Work out the finished part from the listing and answer in its coordinate system (mm). A direction names the side the tool comes from. Coordinates: 2 decimals unless noted, no trailing zeros. Write each loop counter-clockwise with the first axis right and the second up, starting at its lowest first coordinate (ties: lowest second). Pieces come first, ordered by that corner, then holes. Notation, with made-up numbers: M 77,27 L 100,27 A31 ccw 100,65 Z; hole C 78.25,63 d8. An arc over 180 degrees is marked long. Use CSV: the item, a comma, the result in double quotes.
from build123d import *

# Parameters (mm, degrees)
F1_R     = 6.15
F2_DEPTH = 35.5
F3_DEPTH = 35.501
F4_DEPTH = 2
F5_R     = 0.5


# Not quite as in the source:
# - two fillets or chamfers of one size are made in one step


with BuildPart() as f2:
    # F1 (on face) → F2 (new body)
    with BuildSketch(Plane.XZ):
        Circle(F1_R)
    extrude(amount=F2_DEPTH)


with BuildPart() as f2b:
    # F0 (on Front) → F2, piece 2 (new body)
    with BuildSketch(Plane.XZ):
        with BuildLine():
            ThreePointArc((11.8124997243, -2.1130192291), (11.9530330187, -1.0606609515), (12, 0))
            ThreePointArc((12, 0), (-1.0606609515, 11.9530330187), (-11.8124997243, -2.1130192291))
            Line((-11.8124997243, -2.1130192291), (-11.8124997243, 1))
            Line((-11.8124997243, 1), (11.8124997243, 1))
            Line((11.8124997243, 1), (11.8124997243, -2.1130192291))
        make_face()
        with BuildLine():
            Line((-11.8124997243, 1), (-11.8124997243, -2.1130192291))
            ThreePointArc((-11.8124997243, -2.1130192291), (0, -12), (11.8124997243, -2.1130192291))
            Line((11.8124997243, -2.1130192291), (11.8124997243, 1))
            Line((11.8124997243, 1), (-11.8124997243, 1))
        make_face()
        with BuildLine():
            ThreePointArc((11.8124997243, -2.1130192291), (0, -12), (-11.8124997243, -2.1130192291))
            Line((-11.8124997243, -2.1130192291), (-11.8124997243, -13))
            Line((-11.8124997243, -13), (11.8124997243, -13))
            Line((11.8124997243, -13), (11.8124997243, -2.1130192291))
        make_face()
    extrude(amount=F2_DEPTH)


with BuildPart() as f3_tool:
    # F3 (cut, through all): a face of the model
    f3_faces = [f2.part.faces().sort_by_distance(p)[0] for p in [
        (0, -35.5, 0),
    ]]
    extrude(f3_faces, amount=-F3_DEPTH)


with BuildPart() as f2_1:
    add(f2.part)

    # F3: cut by f3_tool
    add(f3_tool.part, mode=Mode.SUBTRACT)


with BuildPart() as f2b_1:
    add(f2b.part)

    # F3: cut by f3_tool
    add(f3_tool.part, mode=Mode.SUBTRACT)

    # F4 (add): a face of the model
    f4_faces = [f2b_1.faces().sort_by_distance(p)[0] for p in [
        (0, -17.75, -13),
    ]]
    extrude(f4_faces, amount=F4_DEPTH)

    # F5
    f5_edges = [f2b_1.edges().sort_by_distance(p)[0] for p in [
        (0, -35.5, 12),
        (-11.8125, -35.5, -8.55651),
        (11.8125, -35.5, -8.55651),
        (11.8125, 0, -8.55651),
        (-11.8125, 0, -8.55651),
        (0, 0, 12),
        (-11.8125, -17.75, -15),
        (0, 0, -15),
        (11.8125, -17.75, -15),
        (0, -35.5, -15),
    ]]
    fillet(f5_edges, radius=F5_R)


solid = f2b_1.part
Item 1: The part is cut by section A-A (y = -13.5). Write down the section's boundary in (x, z), then the cut area to 3 significant figures.
Answer:
outline,"M -11.81,-14.5 A0.5 ccw -11.31,-15 L 11.31,-15 A0.5 ccw 11.81,-14.5 L 11.81,-2.11 A12 ccw long -11.81,-2.11 Z; hole C 0,0 d12.3"
area,"462 mm2"
Item 2: For a pull along Z with two mould halves and no side action, classify faces 4 (the face through (0, -18, -15)), 5 (the face through (0, -35.5, -7)), 6 (the face through (-1.333, -17.998, -6.004)) as released by +Z, released by -Z, zero draft, split by the parting line, or undercut.
Answer:
face 4,"released by -Z"
face 5,"zero draft"
face 6,"undercut"
Item 3: Consider probe 1 along Z at (x, y) = (0, -18); probe 2 along Z at (x, y) = (-3.5, -15.5); probe 3 along X at (y, z) = (-3, -12.75). Determine where each line is inside the solid, lowest interval first.
Answer:
probe 1,"z = -15 to -6.15, 6.15 to 12"
probe 2,"z = -15 to -5.06, 5.06 to 11.48"
probe 3,"x = -11.81 to 11.81"
Item 4: The part is cut by section B-B (z = -7). Write down the section's boundary in (x, y), then the cut area to 3 significant figures.
Answer:
outline,"M -11.81,-35 A0.5 ccw -11.31,-35.5 L 11.31,-35.5 A0.5 ccw 11.81,-35 L 11.81,-0.5 A0.5 ccw 11.31,0 L -11.31,0 A0.5 ccw -11.81,-0.5 Z"
area,"838 mm2"
Item 5: A tool of negligible diameter and unlimited length cuts with its end or side. For faces 1 (the face through (-11.812, -18, -8)), 2 (the face through (0, 0, -7)), 3 (the face through (11.812, -18, -8)), from which of +Z, -Z, +X, -X, +Y, -Y can it reach the whole face along a straight path? Write none if from no direction.
Answer:
face 1,"-Z, -X, +Y, -Y"
face 2,"+Z, -Z, +X, -X, +Y"
face 3,"-Z, +X, +Y, -Y"
Item 6: Given pin 1 (12 mm diameter, centred on x = 1, y = -17.5, fed in from +Z); pin 2 (10 mm diameter, centred on x = 0, z = 0, fed in from +Y); pin 3 (1 mm diameter, centred on y = -30.5, z = -10, fed in from +X); pin 4 (10 mm diameter, centred on y = -17.5, z = -10.5, fed in from -X), each flat-ended and moving along its own axis, determine where each tip first touches the part or whether it passes through.
Answer:
pin 1,"stops at z = 12"
pin 2,"passes through"
pin 3,"stops at x = 11.81"
pin 4,"stops at x = -11.81"
